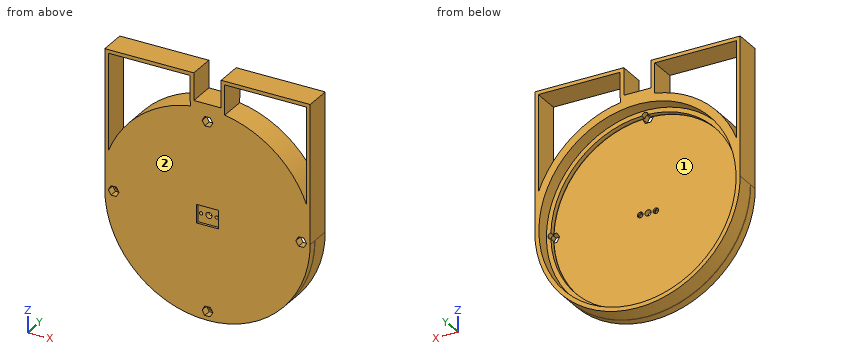
from build123d import *

# Parameters (mm, degrees)
SKETCH073_R     = 57.5
SKETCH073_R_2   = 50.2
PAD023_DEPTH    = 10
SKETCH074_R     = 57.5
SKETCH074_R_2   = 52.7
PAD024_DEPTH    = 10
SKETCH075_R     = 55.2
SKETCH075_R_2   = 45.630592
POCKET038_DEPTH = 10.001
SKETCH076_R     = 55.2
SKETCH076_R_2   = 52.7
PAD025_DEPTH    = 2.6
SKETCH077_R     = 57.5
SKETCH077_R_2   = 52.7
PAD026_DEPTH    = 0.4
SKETCH078_R     = 1.75
POCKET039_DEPTH = 5
SKETCH079_R     = 57.5
PAD027_DEPTH    = 4.4
SKETCH080_W     = 12.18
SKETCH080_H     = 10.29
POCKET040_DEPTH = 1.4
SKETCH081_R     = 1.7
POCKET041_DEPTH = 14.801
SKETCH082_R     = 0.9
POCKET042_DEPTH = 14.801
SKETCH083_R     = 1.55
POCKET043_DEPTH = 1
PAD028_DEPTH    = 14.8


with BuildPart() as part:
    # Sketch073 (on DatumPlane) → Pad023 (new body)
    with BuildSketch(Plane.XZ.offset(10)):
        Circle(SKETCH073_R)
        Circle(SKETCH073_R_2, mode=Mode.SUBTRACT)
    extrude(amount=-PAD023_DEPTH)

    # Sketch074 (on DatumPlane) → Pad024 (new body)
    with BuildSketch(Plane.XZ.offset(10)):
        Circle(SKETCH074_R)
        Circle(SKETCH074_R_2, mode=Mode.SUBTRACT)
    extrude(amount=-PAD024_DEPTH)

    # Sketch075 (on Face4 of PolarPattern008) → Pocket038 (cut, through all)
    with BuildSketch(Plane.XZ.offset(10)):
        Circle(SKETCH075_R)
        Circle(SKETCH075_R_2, mode=Mode.SUBTRACT)
    extrude(amount=-POCKET038_DEPTH, mode=Mode.SUBTRACT)

    # Sketch076 (on Face2 of Pocket038) → Pad025 (new body)
    with BuildSketch(Plane.XZ.offset(10)):
        Circle(SKETCH076_R)
        Circle(SKETCH076_R_2, mode=Mode.SUBTRACT)
    extrude(amount=-PAD025_DEPTH)

    # Sketch077 (on Face6 of Pad025) → Pad026 (new body)
    with BuildSketch(Plane.XZ.offset(10)):
        Circle(SKETCH077_R)
        Circle(SKETCH077_R_2, mode=Mode.SUBTRACT)
    extrude(amount=PAD026_DEPTH)

    # Sketch078 (on Face5 of Pad026) → Pocket039 (cut)
    with BuildSketch(Plane.XZ.offset(10.4)):
        with Locations((0, -52.5)):
            Circle(SKETCH078_R)
        with Locations((-52.5, 0)):
            Circle(SKETCH078_R)
        with Locations((0, 52.5)):
            Circle(SKETCH078_R)
        with Locations((52.5, 0)):
            Circle(SKETCH078_R)
    extrude(amount=-POCKET039_DEPTH, mode=Mode.SUBTRACT)

    # Sketch079 (on Face4 of Pocket039) → Pad027 (new body)
    with BuildSketch(Plane.XZ.offset(10.4)):
        Circle(SKETCH079_R)
        Polygon((3, -52.5), (1.5, -49.901924), (-1.5, -49.901924), (-3, -52.5), (-1.5, -55.098076), (1.5, -55.098076), align=None, mode=Mode.SUBTRACT)
        Polygon((3, 52.5), (1.5, 55.098076), (-1.5, 55.098076), (-3, 52.5), (-1.5, 49.901924), (1.5, 49.901924), align=None, mode=Mode.SUBTRACT)
        Polygon((-49.5, 0), (-51, 2.598076), (-54, 2.598076), (-55.5, 0), (-54, -2.598076), (-51, -2.598076), align=None, mode=Mode.SUBTRACT)
        Polygon((55.5, 0), (54, 2.598076), (51, 2.598076), (49.5, 0), (51, -2.598076), (54, -2.598076), align=None, mode=Mode.SUBTRACT)
    extrude(amount=PAD027_DEPTH)

    # Sketch080 (on Face13 of Pad027) → Pocket040 (cut)
    with BuildSketch(Plane.XZ.offset(14.8)):
        Rectangle(SKETCH080_W, SKETCH080_H)
    extrude(amount=-POCKET040_DEPTH, mode=Mode.SUBTRACT)

    # Sketch081 (on Face4 of Pocket040) → Pocket041 (cut, through all)
    with BuildSketch(Plane.XZ.offset(14.8)):
        Circle(SKETCH081_R)
    extrude(amount=-POCKET041_DEPTH, mode=Mode.SUBTRACT)

    # Sketch082 (on Face4 of Pocket041) → Pocket042 (cut, through all)
    with BuildSketch(Plane.XZ.offset(14.8)):
        with Locations((-4.35, 0)):
            Circle(SKETCH082_R)
        with Locations((4.35, 0)):
            Circle(SKETCH082_R)
    extrude(amount=-POCKET042_DEPTH, mode=Mode.SUBTRACT)

    # Sketch083 (on Face42 of Pocket042) → Pocket043 (cut)
    with BuildSketch(Plane(origin=(0, -10.4, 0), x_dir=(1, 0, 0), z_dir=(0, 1, 0))):
        with Locations((-4.35, 0)):
            Circle(SKETCH083_R)
        with Locations((4.35, 0)):
            Circle(SKETCH083_R)
    extrude(amount=-POCKET043_DEPTH, mode=Mode.SUBTRACT)

    # Sketch084 (on Face1 of Pocket043) → Pad028 (new body)
    with BuildSketch(Plane(origin=(0, 0, 0), x_dir=(1, 0, 0), z_dir=(0, 1, 0))):
        with BuildLine():
            Line((-7.65, -62.26), (7.65, -62.26))
            Line((7.65, -62.26), (7.65, -77.56))
            Line((7.65, -77.56), (57.5, -77.56))
            Line((57.5, 0), (57.5, -77.56))
            ThreePointArc((-57.5, 0), (0, -57.5), (57.5, 0))
            Line((-57.5, 0), (-57.5, -77.56))
            Line((-57.5, -77.56), (-7.65, -77.56))
            Line((-7.65, -62.26), (-7.65, -77.56))
        make_face()
        with BuildLine():
            Line((9.640661, -58.760865), (9.65, -75.56))
            Line((9.65, -75.56), (55.5, -75.56))
            Line((55.500076, -21.447651), (55.5, -75.56))
            ThreePointArc((9.640661, -58.760865), (37.533805, -46.204517), (55.500076, -21.447651))
        make_face(mode=Mode.SUBTRACT)
        with BuildLine():
            Line((-9.65, -75.56), (-55.5, -75.56))
            Line((-55.500076, -21.447651), (-55.5, -75.56))
            ThreePointArc((-55.500076, -21.447651), (-37.533805, -46.204517), (-9.640661, -58.760865))
            Line((-9.640661, -58.760865), (-9.65, -75.56))
        make_face(mode=Mode.SUBTRACT)
    extrude(amount=-PAD028_DEPTH)


solid = part.part
Model file for the job. Use its own axes, mm. Face numbers are marked on the shaded views. Round coordinates to 2 decimals unless told otherwise and drop trailing zeros. Loops run counter-clockwise (first coordinate to the right, second up) from the corner with the lowest first, then second, coordinate; pieces in that order, holes last.
1. Band-saw the part on B-B, the plane y = -5.5. List the corners of the cut face in (x, z).
Check values:
outline: (-57.5, 0) arc R57.5 ccw to (57.5, 0) - (57.5, 77.56) - (7.65, 77.56) - (7.65, 62.26) - (-7.65, 62.26) - (-7.65, 77.56) - (-57.5, 77.56) - close; hole (-55.5, 21.45) arc R59.49 cw to (-9.64, 58.76) - (-9.65, 75.56) - (-55.5, 75.56) - close; hole circle Ø110.4 at (0, 0); hole (9.64, 58.76) arc R59.49 cw to (55.5, 21.45) - (55.5, 75.56) - (9.65, 75.56) - close
2. Drop flat-ended pins along their axis: P1, Ø7.5, axis at x = -40, y = -8.5, coming from the -Z side; P2, Ø0.7, axis at x = 1, z = 54.5, coming from the -Y side; P3, Ø4, axis at x = -24.5, z = 45, coming from the +Y side. Give the stop position or say it passes through.
Check values:
P1: stops at z = -44.63
P2: stops at y = -10.4
P3: stops at y = -7.4
3. Band-saw the part on A-A, the plane x = 0. List the corners of the cut face in (y, z) (3 decimals), and give its area (3 significant figures).
Check values:
outline: (-14.8, -57.5) - (0, -57.5) - (0, -55.2) - (-7.4, -55.2) - (-7.4, -54.25) - (-10.4, -54.25) - (-10.4, -55.098) - (-14.8, -55.098) - close; (-14.8, -49.902) - (-10.4, -49.902) - (-10.4, -1.7) - (-13.4, -1.7) - (-13.4, -5.145) - (-14.8, -5.145) - close; (-14.8, 5.145) - (-13.4, 5.145) - (-13.4, 1.7) - (-10.4, 1.7) - (-10.4, 49.902) - (-14.8, 49.902) - close; (-14.8, 55.098) - (-10.4, 55.098) - (-10.4, 54.25) - (-7.4, 54.25) - (-7.4, 55.2) - (0, 55.2) - (0, 62.26) - (-14.8, 62.26) - close
area: 560 mm2
4. Wall check: probe 1 along Z at (x, y) = (0, -1.75); probe 2 along X at (y, z) = (-3.75, 63); probe 3 along Z at (x, y) = (0, -12.35). Give the ranges that are in metal, low to high.
Check values:
probe 1: z = -57.5 to -55.2, 55.2 to 62.26
probe 2: x = -57.5 to -55.5, -9.64 to -7.65, 7.65 to 9.64, 55.5 to 57.5
probe 3: z = -57.5 to -55.1, -49.9 to -1.7, 1.7 to 49.9, 55.1 to 62.26
5. Band-saw the part on C-C, the plane z = 48. List the corners of the cut face in (x, y).
Check values:
outline: (-57.5, -14.8) - (-55.5, -14.8) - (-55.5, 0) - (-57.5, 0) - close; (-35.21, -14.8) - (35.21, -14.8) - (35.21, 0) - (27.26, 0) - (27.26, -7.4) - (21.76, -7.4) - (21.76, -10.4) - (-21.76, -10.4) - (-21.76, -7.4) - (-27.26, -7.4) - (-27.26, 0) - (-35.21, 0) - close; (55.5, -14.8) - (57.5, -14.8) - (57.5, 0) - (55.5, 0) - close
6. Mould opens along X. For the marked faces 1 and 2 say: +X half, -X half, draft (parallel to the pull), parting line (faces both ways), or undercut.
Check values:
face 1: undercut
face 2: draft
7. Band-saw the part on D-D, the plane x = -26.5. List the corners of the cut face in (y, z), and give its area (3 significant figures).
Check values:
outline: (-14.8, -51.03) - (0, -51.03) - (0, -48.42) - (-7.4, -48.42) - (-7.4, -45.55) - (-10.4, -45.55) - (-10.4, 45.55) - (-7.4, 45.55) - (-7.4, 48.42) - (0, 48.42) - (0, 53.32) - (-14.8, 53.32) - close; (-14.8, 75.56) - (0, 75.56) - (0, 77.56) - (-14.8, 77.56) - close
area: 584 mm2
